Source: CAD feature listing. Evaluate the final solid. Frame: model axes, mm. Round coordinates to 2 decimals unless told otherwise and drop trailing zeros. Order: outer loops, then holes, each group sorted by start corner. A loop starts at its lowest first (then second) coordinate and runs counter-clockwise, first axis right, second up. Notation, with made-up numbers: (49, 52) -> (91, 52) arc R8 ccw to (91, 62) -> close; hole circle Ø10 at (60.5, 64.25). An arc over 180 degrees is marked (long way). Answer as CSV lines item,"result". Start each with the question number.
(1) Section query B-B (z = 0). Output: boundary loops of the cut face in (x, y) (1 decimal), plus the area to 3 significant figures.
(2) Pull-direction query (X, two-part tool) for faces 1 (the flat face through (-10, 2, -4.762)), 2 (the cylindrical face through (-9, 1.6, -1.5)), 3 (the cylindrical face through (1.285, 1.565, -0.819)), 4 (the flat face through (-27.287, 1.252, 0.067)); classes: +X half, -X half, draft (parallel to the pull), parting line (faces both ways), or undercut.
(3) Line query: line 1 along X through (y, z) = (1.1, 0) (1 decimal); line 2 along X through (y, z) = (1.8, 0) (1 decimal); line 3 along Z through (x, y) = (-0.5, 1.05). Output: solid intervals per line, ascending. Write a range as from..to.
(4) Section query D-D (z = 2.5). Output: boundary loops of the cut face in (x, y) (3 decimals).
(5) Section query A-A (x = 0). Output: boundary loops of the cut face in (y, z) (1 decimal).
(6) Section query C-C (y = 0.35). Count the separate pieces of the cut face and the enclosed holes in it, plus the area to 3 significant figures.
```python
from build123d import *

# Parameters (mm, degrees)
SKETCH1_W           = 38.1
SKETCH1_H           = 9.525
BOSS_EXTRUDE1_DEPTH = 3.175
SKETCH2_R           = 1.651
SKETCH2_R_2         = 1.5875
SKETCH2_R_3         = 1.524
CUT_EXTRUDE1_DEPTH  = 30.142626104
CHAMFER1_SIZE       = 2.54


with BuildPart() as part:
    # Sketch1 → Boss-Extrude1 (new body)
    with BuildSketch(Plane(origin=(0, 0, 0), x_dir=(1, 0, 0), z_dir=(0, 1, 0))):
        with Locations((-9.525, 0)):
            Rectangle(SKETCH1_W, SKETCH1_H)
    extrude(amount=BOSS_EXTRUDE1_DEPTH)

    # Sketch2 → Cut-Extrude1 (cut, through all)
    with BuildSketch(Plane.XZ):
        with Locations(Location((-19.05, 0, 0), (0, 0, 270))):
            Circle(SKETCH2_R)
        with Locations(Location((-9.525, 0, 0), (0, 0, 270))):
            Circle(SKETCH2_R_2)
        with Locations(Location((0, 0, 0), (0, 0, 270))):
            Circle(SKETCH2_R_3)
    extrude(amount=-CUT_EXTRUDE1_DEPTH, mode=Mode.SUBTRACT)

    # Chamfer1
    chamfer1_edges = [part.edges().sort_by_distance(p)[0] for p in [
        (-28.575, 0, 0),
    ]]
    chamfer(chamfer1_edges, length=CHAMFER1_SIZE)


solid = part.part
```
Answer block:
1,outline,"(-28.6, 2.5) -> (-26, 0) -> (-20.7, 0) -> (-20.7, 3.2) -> (-28.6, 3.2) -> close; (-17.4, 0) -> (-11.1, 0) -> (-11.1, 3.2) -> (-17.4, 3.2) -> close; (-7.9, 0) -> (-1.5, 0) -> (-1.5, 3.2) -> (-7.9, 3.2) -> close; (1.5, 0) -> (9.5, 0) -> (9.5, 3.2) -> (1.5, 3.2) -> close"
1,area,"87.5 mm2"
2,face 1,"draft"
2,face 2,"undercut"
2,face 3,"undercut"
2,face 4,"-X half"
3,line 1,"-27.1..-20.7, -17.4..-11.1, -7.9..-1.5, 1.5..9.5"
3,line 2,"-27.8..-20.7, -17.4..-11.1, -7.9..-1.5, 1.5..9.5"
3,line 3,"-4.76..-1.44, 1.44..4.76"
4,outline,"(-28.575, 2.54) -> (-26.035, 0) -> (9.525, 0) -> (9.525, 3.175) -> (-28.575, 3.175) -> close"
5,outline,"(0, -4.8) -> (3.2, -4.8) -> (3.2, -1.5) -> (0, -1.5) -> close; (0, 1.5) -> (3.2, 1.5) -> (3.2, 4.8) -> (0, 4.8) -> close"
6,separate pieces,"1"
6,enclosed holes,"3"
6,area,"318 mm2"
